The model under review builds one solid part; all positions refer to its coordinate system, in mm. A direction names the side the tool comes from. Coordinates: 2 decimals unless noted, no trailing zeros. Return JSON: item names as keys, results as strings.
```python
from build123d import *

# Parameters (mm, degrees)
SKETCH2_R           = 115
BOSS_EXTRUDE1_DEPTH = 25
SKETCH3_R           = 85
CUT_EXTRUDE1_DEPTH  = 16
SKETCH4_R           = 83
CUT_EXTRUDE2_DEPTH  = 164.419705054
CHAMFER3_SIZE       = 2
CHAMFER5_SIZE       = 1
FILLET1_R           = 3
SKETCH5_R           = 4
CUT_EXTRUDE3_DEPTH  = 15
SKETCH6_R           = 6
CUT_EXTRUDE4_DEPTH  = 10
CHAMFER6_SIZE       = 1


with BuildPart() as part:
    # Sketch2 → Boss-Extrude1 (new body)
    with BuildSketch(Plane(origin=(0, 0, 0), x_dir=(1, 0, 0), z_dir=(0, 1, 0))):
        with Locations(Location((0, 0, 0), (0, 0, 270))):
            Circle(SKETCH2_R)
    extrude(amount=BOSS_EXTRUDE1_DEPTH)

    # Sketch3 → Cut-Extrude1 (cut)
    with BuildSketch(Plane(origin=(0, 25, 0), x_dir=(1, 0, 0), z_dir=(0, 1, 0))):
        with Locations(Location((0, 0, 0), (0, 0, 270))):
            Circle(SKETCH3_R)
    extrude(amount=-CUT_EXTRUDE1_DEPTH, mode=Mode.SUBTRACT)

    # Sketch4 → Cut-Extrude2 (cut, through all)
    with BuildSketch(Plane(origin=(0, 9, 0), x_dir=(1, 0, 0), z_dir=(0, 1, 0))):
        with Locations(Location((0, 0, 0), (0, 0, 270))):
            Circle(SKETCH4_R)
    extrude(amount=-CUT_EXTRUDE2_DEPTH, mode=Mode.SUBTRACT)

    # Chamfer3
    chamfer3_edges = [part.edges().sort_by_distance(p)[0] for p in [
        (0, 9, -85),
    ]]
    chamfer(chamfer3_edges, length=CHAMFER3_SIZE - 0.0001)  # a hair under: the kernel refuses the full size

    # Chamfer5
    chamfer5_edges = [part.edges().sort_by_distance(p)[0] for p in [
        (0, 25, -115),
        (0, 25, -85),
    ]]
    chamfer(chamfer5_edges, length=CHAMFER5_SIZE)

    # Fillet1
    fillet1_edges = [part.edges().sort_by_distance(p)[0] for p in [
        (0, 0, -83),
        (0, 0, -115),
    ]]
    fillet(fillet1_edges, radius=FILLET1_R)

    # Sketch5 → Cut-Extrude3 (cut)
    with BuildSketch(Plane(origin=(0, 25, 0), x_dir=(1, 0, 0), z_dir=(0, 1, 0))):
        with Locations(Location((-100, 0, 0), (0, 0, 270))):
            Circle(SKETCH5_R)
        with Locations(Location((-70.710678119, 70.710678119, 0), (0, 0, 270))):
            Circle(SKETCH5_R)
        with Locations(Location((0, 100, 0), (0, 0, 270))):
            Circle(SKETCH5_R)
        with Locations(Location((70.710678119, 70.710678119, 0), (0, 0, 270))):
            Circle(SKETCH5_R)
        with Locations(Location((100, 0, 0), (0, 0, 270))):
            Circle(SKETCH5_R)
        with Locations(Location((70.710678119, -70.710678119, 0), (0, 0, 270))):
            Circle(SKETCH5_R)
        with Locations(Location((0, -100, 0), (0, 0, 270))):
            Circle(SKETCH5_R)
        with Locations(Location((-70.710678119, -70.710678119, 0), (0, 0, 270))):
            Circle(SKETCH5_R)
    extrude(amount=-CUT_EXTRUDE3_DEPTH, mode=Mode.SUBTRACT)

    # Sketch6 → Cut-Extrude4 (cut)
    with BuildSketch(Plane.XZ):
        with Locations(Location((-100, 0, 0), (0, 0, 270))):
            Circle(SKETCH6_R)
        with Locations(Location((-70.710678119, 70.710678119, 0), (0, 0, 270))):
            Circle(SKETCH6_R)
        with Locations(Location((0, 100, 0), (0, 0, 270))):
            Circle(SKETCH6_R)
        with Locations(Location((70.710678119, 70.710678119, 0), (0, 0, 270))):
            Circle(SKETCH6_R)
        with Locations(Location((100, 0, 0), (0, 0, 270))):
            Circle(SKETCH6_R)
        with Locations(Location((70.710678119, -70.710678119, 0), (0, 0, 270))):
            Circle(SKETCH6_R)
        with Locations(Location((0, -100, 0), (0, 0, 270))):
            Circle(SKETCH6_R)
        with Locations(Location((-70.710678119, -70.710678119, 0), (0, 0, 270))):
            Circle(SKETCH6_R)
    extrude(amount=-CUT_EXTRUDE4_DEPTH, mode=Mode.SUBTRACT)

    # Chamfer6
    chamfer6_edges = [part.edges().sort_by_distance(p)[0] for p in [
        (-100, 25, -4),
        (-70.710678119, 25, -74.710678119),
        (0, 25, -104),
        (70.710678119, 25, -74.710678119),
        (100, 25, -4),
        (70.710678119, 25, 66.710678119),
        (0, 25, 96),
        (-70.710678119, 25, 66.710678119),
    ]]
    chamfer(chamfer6_edges, length=CHAMFER6_SIZE)


solid = part.part
```
1. Add section A-A on z = 0. State how many separate pieces and enclosed holes the cut face has, plus the area to 3 significant figures.
Check values:
{"separate pieces": "4", "enclosed holes": "0", "area": "1,050 mm²"}
2. Insertion check: pin 1 Ø6 at (x, z) = (-73.5, -70.5) entering from -Y; pin 2 Ø12 at (y, z) = (11.5, 70) entering from -X; pin 3 Ø9.5 at (x, z) = (-70.71, 70.71) entering from +Y. Each pin has a flat end and moves straight along its axis. Give the tip position at first contact, or say it passes through.
Check values:
{"pin 1": "y = 10", "pin 2": "x = -95.55", "pin 3": "y = 24.75"}
3. To check wall thickness, follow line 1 (X direction, y = 6.2, z = 0); line 2 (Z direction, x = -71, y = 10.5); line 3 (Z direction, x = 3, y = 22.25). State the ranges of each line that lie inside material, in increasing order.
Check values:
{"line 1": "-115 to -106, -94 to -83, 83 to 94, 106 to 115", "line 2": "-90.47 to -74.7, -66.72 to -45.82, 45.82 to 66.72, 74.7 to 90.47", "line 3": "-114.96 to -102.65, -97.35 to -84.95, 84.95 to 97.35, 102.65 to 114.96"}
4. The part is to be moulded in two halves that separate along Z. For faces 3 (the face through (72.513, 4.93, -76.434)), 4 (the face through (-112.265, 13.353, -24.93)), say which applies: released by +Z, released by -Z, zero draft, split by the parting line, or undercut.
Check values:
{"face 3": "undercut", "face 4": "split by the parting line"}
5. Machinability: for faces 1 (the face through (0, 5, 106)), 2 (the face through (-72.2, 17.1, -67)), which of the approach directions +Z, -Z, +X, -X, +Y, -Y give a long, thin tool a straight path to every point of the face, cutting with its end or side? Answer none if there is none.
Check values:
{"face 1": "-Y", "face 2": "+Y, -Y"}
